Geometry: final body of the model. Coordinates: model frame, mm. A direction names the side the tool comes from. Round coordinates to 2 decimals unless told otherwise and drop trailing zeros. Write each loop counter-clockwise with the first axis right and the second up, starting at its lowest first coordinate (ties: lowest second). Pieces come first, ordered by that corner, then holes. Notation, with made-up numbers: (7.25, 10) - (36.25, 10) arc R24 cw to (36.25, 26) - close; hole circle Ø10 at (0.5, 22.25). An arc over 180 degrees is marked (long way). Use a Markdown table: item, result. Add a question column.
```python
from build123d import *

# Parameters (mm, degrees)
SKETCH1_R           = 1.8
BOSS_EXTRUDE1_DEPTH = 2.5
BOSS_EXTRUDE2_START = 2.5
SKETCH1_4_R         = 1.8
BOSS_EXTRUDE2_DEPTH = 5
CHAMFER1_SIZE       = 1
CHAMFER2_SIZE       = 0.5


with BuildPart() as part:
    # Sketch1 → Boss-Extrude1 (new body)
    with BuildSketch(Plane(origin=(0, 0, 0), x_dir=(1, 0, 0), z_dir=(0, 1, 0))):
        with BuildLine():
            Line((0, -11.62), (0, -3.62))
            ThreePointArc((0, -3.62), (-2.559726548, -2.559726548), (-3.62, 0))
            Line((-3.62, 0), (-3.62, 17.18))
            Line((-3.62, 17.18), (-11.9, 17.18))
            Line((-11.9, 17.18), (-11.9, -5.717458175))
            Line((-11.9, -5.717458175), (-6.5, -11.62))
            Line((-6.5, -11.62), (0, -11.62))
        make_face()
        with Locations((-3.25, -7.42)):
            Circle(SKETCH1_R, mode=Mode.SUBTRACT)
        with BuildLine():
            ThreePointArc((-9.9, -2.82), (-7.76, -4.96), (-5.62, -2.82))
            Line((-5.62, -2.82), (-5.62, 12.68))
            ThreePointArc((-5.62, 12.68), (-7.76, 14.82), (-9.9, 12.68))
            Line((-9.9, 12.68), (-9.9, -2.82))
        make_face(mode=Mode.SUBTRACT)
        with Locations((-3.25, -7.42)):
            Circle(SKETCH1_R)
    extrude(amount=BOSS_EXTRUDE1_DEPTH)

    # Sketch1<4> → Boss-Extrude2 (add)
    with BuildSketch(Plane(origin=(0, 0, 0), x_dir=(1, 0, 0), z_dir=(0, 1, 0)).offset(BOSS_EXTRUDE2_START)):
        with BuildLine():
            Line((-3.62, 0), (-3.62, 17.18))
            Line((-3.62, 17.18), (-11.9, 17.18))
            Line((-11.9, 17.18), (-11.9, -5.717458175))
            Line((-11.9, -5.717458175), (-6.5, -11.62))
            Line((-6.5, -11.62), (0, -11.62))
            Line((0, -11.62), (0, -3.62))
            ThreePointArc((0, -3.62), (-2.559726548, -2.559726548), (-3.62, 0))
        make_face()
        with Locations(Location((-3.25, -7.42, 0), (0, 0, 270))):
            Circle(SKETCH1_4_R, mode=Mode.SUBTRACT)
        with BuildLine():
            Line((-5.62, 12.68), (-5.62, -2.82))
            ThreePointArc((-5.62, -2.82), (-7.76, -4.96), (-9.9, -2.82))
            Line((-9.9, -2.82), (-9.9, 12.68))
            ThreePointArc((-9.9, 12.68), (-7.76, 14.82), (-5.62, 12.68))
        make_face(mode=Mode.SUBTRACT)
    extrude(amount=BOSS_EXTRUDE2_DEPTH)

    # Chamfer1
    chamfer1_edges = [part.edges().sort_by_distance(p)[0] for p in [
        (-3.25, 0, 11.62),
        (-9.2, 0, 8.668729087),
        (-11.9, 0, -5.731270913),
        (-7.76, 0, -17.18),
        (-3.62, 0, -8.59),
        (-2.559726548, 0, 2.559726548),
        (-11.9, 3.75, -17.18),
        (-3.62, 3.75, -17.18),
        (-2.559726548, 7.5, 2.559726548),
        (-3.62, 7.5, -8.59),
        (-7.76, 7.5, -17.18),
        (-11.9, 7.5, -5.731270913),
        (-9.2, 7.5, 8.668729087),
        (-3.25, 7.5, 11.62),
    ]]
    chamfer(chamfer1_edges, length=CHAMFER1_SIZE)

    # Chamfer2
    chamfer2_edges = [part.edges().sort_by_distance(p)[0] for p in [
        (-5.62, 0, -4.93),
        (-7.76, 0, -14.82),
        (-9.9, 0, -4.93),
        (-7.76, 0, 4.96),
        (-5.62, 7.5, -4.93),
        (-9.9, 7.5, -4.93),
        (-7.76, 7.5, 4.96),
        (-7.76, 7.5, -14.82),
        (-3.25, 7.5, 5.62),
    ]]
    chamfer(chamfer2_edges, length=CHAMFER2_SIZE)

    # Mirror1: part across plane


with BuildPart() as part_1:
    add(part.part)
    add(part.part.mirror(Plane(origin=(0, 2.5, 0), x_dir=(0, 0, 1), z_dir=(-1, 0, 0))))


solid = part_1.part
```
1) Section B-B, the plane z = -8.25. State how many separate pieces and enclosed holes the cut face has, then the cut area to 3 significant figures.
2) Set-up query: faces 5 (the conical face through (-7.81, 7.135, -14.955)), 6 (the flat face through (4.11, 6.99, -7.98)), 7 (the cylindrical face through (7.81, 3.7, -14.82)). Return all of +Z, -Z, +X, -X, +Y, -Y with unobstructed straight access to the full face (end or side cutting, diameter ignored); none if empty.
3) Section C-C, the plane z = 7.42. Return the cut outline in (x, y), then the cut area to 3 significant figures.
4) Material intervals for L1, parallel to X at y = 4, z = -4.5; L2, parallel to X at y = 2.75, z = 3.75; L3, parallel to X at y = 3.9, z = 7.42, sorted ascending. Write a range as from..to.
5) Pin query (flat end, axial travel): P1, Ø1.8, axis at x = 4, z = 7.5, coming from the +Y side; P2, Ø5, axis at x = -9.5, z = 3, coming from the -Y side; P3, Ø3, axis at x = 1.5, z = 2.5, coming from the -Y side. Return the tip coordinate at first contact, or that it passes through.
6) Section A-A, the plane y = 4. Return the cut outline in (x, z).
7) Draft query along Z for faces 1 (the flat face through (9.9, 4, -5)), 2 (the flat face through (0, 4, 11.62)), 3 (the flat face through (-11.39, 3.71, -16.69)), 4 (the flat face through (-9.9, 4, -5)). Return one class per face: released by +Z, released by -Z, zero draft, split by the parting line, or undercut.
Output values:
| question | item | result |
|---|---|---|
| 1 | separate pieces | 4 |
| 1 | enclosed holes | 0 |
| 1 | area | 55.0 mm^2 |
| 2 | face 5 | +Y |
| 2 | face 6 | -Z, +Y |
| 2 | face 7 | +Y, -Y |
| 3 | outline | (-10.34, 1) - (-8.99, 0) - (8.99, 0) - (10.34, 1) - (10.34, 6.5) - (8.99, 7.5) - (5.55, 7.5) - (5.05, 7) - (5.05, 2.5) - (1.45, 2.5) - (1.45, 7) - (0.95, 7.5) - (-0.95, 7.5) - (-1.45, 7) - (-1.45, 2.5) - (-5.05, 2.5) - (-5.05, 7) - (-5.55, 7.5) - (-8.99, 7.5) - (-10.34, 6.5) - close |
| 3 | area | 116 mm^2 |
| 4 | L1 | x = -11.9..-9.9, -5.62..-3.62, 3.62..5.62, 9.9..11.9 |
| 4 | L2 | x = -11.9..-9.69, -5.83..5.83, 9.69..11.9 |
| 4 | L3 | x = -10.34..-5.05, -1.45..1.45, 5.05..10.34 |
| 5 | P1 | stops at y = 2.5 |
| 5 | P2 | stops at y = 0 |
| 5 | P3 | stops at y = 0.2 |
| 6 | outline | (-11.9, -16.18) - (-10.9, -17.18) - (-4.62, -17.18) - (-3.62, -16.18) - (-3.62, 0) arc R3.62 cw to (3.62, 0) - (3.62, -16.18) - (4.62, -17.18) - (10.9, -17.18) - (11.9, -16.18) - (11.9, 5.72) - (6.5, 11.62) - (-6.5, 11.62) - (-11.9, 5.72) - close; hole (-9.9, -12.68) arc R2.14 ccw to (-5.62, -12.68) - (-5.62, 2.82) arc R2.14 ccw to (-9.9, 2.82) - close; hole circle Ø3.6 at (-3.25, 7.42); hole circle Ø3.6 at (3.25, 7.42); hole (5.62, -12.68) arc R2.14 ccw to (9.9, -12.68) - (9.9, 2.82) arc R2.14 ccw to (5.62, 2.82) - close |
| 7 | face 1 | undercut |
| 7 | face 2 | released by +Z |
| 7 | face 3 | released by -Z |
| 7 | face 4 | undercut |
